Here's how the part is built. I have some questions about the finished solid (model axes, mm). A direction names the side the tool comes from. Round coordinates to 2 decimals unless told otherwise and drop trailing zeros. Loops run counter-clockwise (first coordinate to the right, second up) from the corner with the lowest first, then second, coordinate; pieces in that order, holes last. Notation, with made-up numbers: (-18, -35) - (20, -35) arc R32 ccw to (20, -1) - close; hole circle Ø9 at (-28.5, 69). An arc over 180 degrees is marked (long way). Return JSON: item names as keys, results as strings. Group by question number.
Solid Edge part; units mm, degrees
sketch "Sketch1" plane through (0, 0, 0) normal (1, 0, 0) x (0, 1, 0)
  line L0 (-13.5, 17.5) -> (-13.5, 15)
  line L1 (-9.2285, 4.3729) -> (-13.5, 15)
  arc A0 (-9.2285, 4.3729) -> (-10.1564, 3) centre (-10.1564, 4) cw
  line L2 (-13.5, 3) -> (-10.1564, 3)
  line L3 (-13.5, 3) -> (-13.5, 0)
  line L4 (-13.5, 0) -> (13.5, 0)
  line L5 (13.5, 0) -> (13.5, 3)
  line L6 (10.16, 3) -> (13.5, 3)
  arc A1 (9.2749, 4.4654) -> (10.16, 3) centre (10.16, 4) ccw
  line L7 (13.5, 12.5) -> (9.2749, 4.4654)
  line L8 (13.5, 12.5) -> (13.5, 15)
  line L9 (13.5, 15) -> (12, 15)
  line L10 (12, 15) -> (12, 13.5)
  line L11 (12, 13.5) -> (10, 13.5)
  line L12 (10, 13.5) -> (10, 19)
  line L13 (10, 19) -> (-9.5, 19)
  line L14 (-9.5, 19) -> (-9.5, 16.5)
  line L15 (-9.5, 16.5) -> (-11.5, 16.5)
  line L16 (-11.5, 16.5) -> (-11.5, 17.5)
  line L17 (-11.5, 17.5) -> (-13.5, 17.5)
revolve "RevolvedProtrusion1" add sketch "Sketch1" angle 360 about axis through (0, -13.5, 0) along (0, 1, 0)
sketch "Sketch2" plane through (0, 0, 0) normal (0, -1, 0) x (1, 0, 0)
  line L0 (-16.5389, 18.0919) -> (-1, 20.5018)
  line L1 (-1, 6.4613) -> (-1, 20.5018)
  arc A0 (-1, 6.4613) -> (-3.7811, 5.3341) centre (0, 0) ccw
  line L2 (-16.5389, 18.0919) -> (-3.7811, 5.3341)
  line L3 (16.5389, 18.0919) -> (1, 20.5018)
  line L4 (1, 6.4613) -> (1, 20.5018)
  arc A1 (1, 6.4613) -> (3.7811, 5.3341) centre (0, 0) cw
  line L5 (16.5389, 18.0919) -> (3.7811, 5.3341)
  line L6 (-17.9531, 16.6777) -> (-5.2168, 3.9413)
  arc A2 (-5.2168, 3.9413) -> (-6.4613, 1) centre (0, 0) ccw
  line L7 (-6.4613, 1) -> (-22.8351, 1)
  line L8 (-17.9531, 16.6777) -> (-22.8351, 1)
  line L9 (17.9531, 16.6777) -> (22.8351, 1)
  line L10 (6.4613, 1) -> (22.8351, 1)
  line L11 (17.9531, 16.6777) -> (5.2168, 3.9413)
  arc A3 (5.2168, 3.9413) -> (6.4614, 1) centre (0, 0) cw
  line L12 (-17.9531, -16.6777) -> (-22.8351, -1)
  line L13 (-6.4613, -1) -> (-22.8351, -1)
  arc A4 (-5.2168, -3.9413) -> (-6.4613, -1) centre (0, 0) cw
  line L14 (-17.9531, -16.6777) -> (-5.2168, -3.9413)
  line L15 (-16.5389, -18.0919) -> (-1, -20.5018)
  line L16 (-1, -6.4613) -> (-1, -20.5018)
  arc A5 (-1, -6.4613) -> (-3.7811, -5.3341) centre (0, 0) cw
  line L17 (-16.5389, -18.0919) -> (-3.7811, -5.3341)
  line L18 (16.5389, -18.0919) -> (3.7811, -5.3341)
  arc A6 (1, -6.4613) -> (3.7811, -5.3341) centre (0, 0) ccw
  line L19 (1, -6.4613) -> (1, -20.5018)
  line L20 (16.5389, -18.0919) -> (1, -20.5018)
  line L21 (17.9531, -16.6777) -> (22.8351, -1)
  line L22 (6.4613, -1) -> (22.8351, -1)
  arc A7 (5.2168, -3.9413) -> (6.4613, -1) centre (0, 0) ccw
  line L23 (17.9531, -16.6777) -> (5.2168, -3.9413)
extrude "VaciadoExtruido_1" cut sketch "Sketch2" along normal blind 8 and the other way blind 8
sketch "Sketch3" plane through (0, 0, 0) normal (0, -1, 0) x (1, 0, 0)
  line L0 (2, -2) -> (-2, -2)
  line L1 (-2, -2) -> (-2, 2)
  line L2 (-2, 2) -> (2, 2)
  line L3 (2, 2) -> (2, -2)
extrude "Cutout1" cut sketch "Sketch3" along normal up to surface (27 mm away) from surface at -13.5
sketch "Sketch4" plane through (-2, 0, 0) normal (1, 0, 0) x (0, 1, 0)
  circle A0 centre (11.5, 0) radius 1.25
extrude "Cutout2" cut sketch "Sketch4" along normal up to next and the other way up to next
Q1. Will these pins go through, and if not, where does the flat tip stop? pin 1 Ø10 at (x, y) = (13.5, 9) entering from -Z; pin 2 Ø6 at (x, z) = (9, -14.5) entering from +Y; pin 3 Ø1.2 at (y, z) = (3, 0) entering from -X; pin 4 Ø6.5 at (x, y) = (-15, 0) entering from -Z.
Q2. Please list where these lines run through material, in increasing order: line 1 (Y direction, x = -2.6, z = 0); line 2 (X direction, y = 7.25, z = -14); line 3 (X direction, y = 10.25, z = 1).
Q3. Imagine slicing it at C-C, the plane x = 16. List the corners of the cut face in (y, z) for me.
Q4. For faces 5 (the flat face through (12, 8, 5)), 6 (the cylindrical face through (0, -12, -3)), 7 (the cylindrical face through (2.48, 0.11, -6.05)), 8 (the cylindrical face through (-6, 0.1, -2.6)), 9 (the flat face through (1, 0, 13)), which set-ups out of +Z, -Z, +X, -X, +Y, -Y let a thin tool reach every point of the face, with its end or its side?
Q5. Imagine slicing it at B-B, the plane z = 0. Give the number of separate pieces and of enclosed holes in the cut face, and give its area (3 significant figures).
Q6. If we mould it in two halves opening along Y, with no side actions, what happens to faces 1 (the flat face through (8, -13.5, 13)), 2 (the flat face through (12, -8, 5)), 3 (the conical face through (-4.85, 9.54, -1.08)), 4 (the flat face through (0, 0, -2))? For each: +Y half, -Y half, draft (parallel to the pull), parting line (faces both ways), or undercut.
Q7. Imagine slicing it at A-A, the plane y = 11.5. List the corners of the cut face in (x, z) for me, and give its area (3 significant figures).
Output values:
{
 "1": {"pin 1": "stops at z = -16.99", "pin 2": "stops at y = 13.5", "pin 3": "stops at x = -19", "pin 4": "stops at z = -14.19"},
 "2": {"line 1": "y = -13.5 to 10.25, 12.75 to 13.5", "line 2": "x = -12.85 to -12.45, -1 to 1, 12.45 to 12.85", "line 3": "x = -13.46 to -6.24, -2.83 to -2, 2 to 2.83, 6.24 to 13.46"},
 "3": {"outline": "(-13.5, -7.09) - (-11.5, -7.09) - (-11.5, -4.03) - (-9.5, -4.03) - (-9.5, -10.25) - (-8, -10.25) - (-8, -1) - (8, -1) - (8, -10.25) - (10, -10.25) - (10, 10.25) - (8, 10.25) - (8, 1) - (-8, 1) - (-8, 10.25) - (-9.5, 10.25) - (-9.5, 4.03) - (-11.5, 4.03) - (-11.5, 7.09) - (-13.5, 7.09) - close"},
 "4": {"face 5": "+X", "face 6": "-Y", "face 7": "-Z", "face 8": "-X", "face 9": "+Z"},
 "5": {"separate pieces": "4", "enclosed holes": "0", "area": "760 mm^2"},
 "6": {"face 1": "-Y half", "face 2": "undercut", "face 3": "+Y half", "face 4": "draft"},
 "7": {"outline": "circle Ø27 at (0, 0); (-2.73, -1.25) arc R3 ccw to (2.73, -1.25) - (2, -1.25) - (2, -2) - (-2, -2) - (-2, -1.25) - close; (-2.73, 1.25) - (-2, 1.25) - (-2, 2) - (2, 2) - (2, 1.25) - (2.73, 1.25) arc R3 ccw to start; hole circle Ø17.39 at (0, 0)", "area": "343 mm^2"}
}
